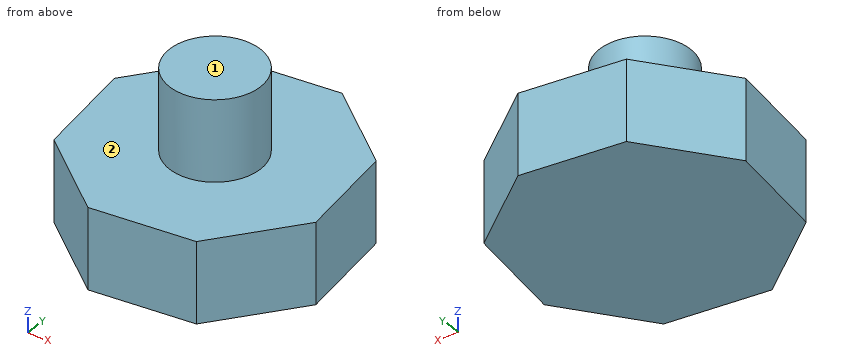
from build123d import *

# Parameters (mm, degrees)
F1_DEPTH = 25.4
F2_R     = 14.326278
F3_DEPTH = 25.4


with BuildPart() as f1:
    # F0 (on Top) → F1 (new body)
    with BuildSketch(Plane.XY):
        Polygon((20.745088, -35.616433), (39.853613, -10.515629), (35.616433, 20.745088), (10.515629, 39.853613), (-20.745088, 35.616433), (-39.853613, 10.515629), (-35.616433, -20.745088), (-10.515629, -39.853613), align=None)
    extrude(amount=F1_DEPTH)

    # F2 (on face) → F3 (join)
    with BuildSketch(Plane.XY.offset(25.4)):
        Circle(F2_R)
    extrude(amount=F3_DEPTH)


solid = f1.part
Work out the finished part from the listing and answer in its coordinate system (mm). Face numbers are marked on the shaded views. A direction names the side the tool comes from. Round coordinates to 2 decimals unless told otherwise and drop trailing zeros. Write each loop counter-clockwise with the first axis right and the second up, starting at its lowest first coordinate (ties: lowest second). Pieces come first, ordered by that corner, then holes.
1) A cutting plane is placed at B-B (x = -3). Give the vertices of the cut face in (y, z).
2) A cutting plane is placed at D-D (z = 31). Give the vertices of the cut face in (x, y).
3) Given pin 1 Ø1 at (y, z) = (-26.5, 14) entering from -X; pin 2 Ø5 at (x, z) = (6, 21) entering from +Y; pin 3 Ø5 at (y, z) = (-10, 25) entering from -X, each flat-ended and moving along its own axis, determine where each tip first touches the part or whether it passes through.
4) A cutting plane is placed at C-C (y = -28.5). Give the vertices of the cut face in (x, z), plus the area to 3 significant figures.
5) A cutting plane is placed at A-A (z = 24). Give the vertices of the cut face in (x, y).
6) A tool of negligible diameter and unlimited length cuts with its end or side. For the marked faces 1 and 2, from which of +Z, -Z, +X, -X, +Y, -Y can it reach the whole face along a straight path? Write none if from no direction.
7) Straight lines are drawn through the part: line 1 (Z direction, x = -17, y = 15.5); line 2 (X direction, y = -14, z = 19.5); line 3 (Y direction, x = -5.5, z = 44.5). For each, find the intervals that lie inside material, in ascending order.
Completed:
1. outline: (-38.83, 0) - (38.02, 0) - (38.02, 25.4) - (14.01, 25.4) - (14.01, 50.8) - (-14.01, 50.8) - (-14.01, 25.4) - (-38.83, 25.4) - close
2. outline: circle Ø28.65 at (0, 0)
3. pin 1: stops at x = -28.71
3. pin 2: stops at y = 39.58
3. pin 3: stops at x = -37.41
4. outline: (-25.43, 0) - (26.16, 0) - (26.16, 25.4) - (-25.43, 25.4) - close
4. area: 1,310 mm2
5. outline: (-39.85, 10.52) - (-35.62, -20.75) - (-10.52, -39.85) - (20.75, -35.62) - (39.85, -10.52) - (35.62, 20.75) - (10.52, 39.85) - (-20.75, 35.62) - close
6. face 1: +Z, +X, -X, +Y, -Y
6. face 2: +Z
7. line 1: z = 0 to 25.4
7. line 2: x = -36.53 to 37.2
7. line 3: y = -13.23 to 13.23
